Input: dimensioned drawing with shaded views. Units: mm. Origin: part minimum x, y, z. Round coordinates to 2 decimals unless told otherwise and drop trailing zeros. Loops run counter-clockwise (first coordinate to the right, second up) from the corner with the lowest first, then second, coordinate; pieces in that order, holes last. Notation, with made-up numbers: (34, -23) - (62, -23) arc R12 cw to (62, -16) - close; hole circle Ø1 at (22, 83). An arc over 180 degrees is marked (long way). Use CSV: the item, a comma, the result in double quotes. Start each with the question number.
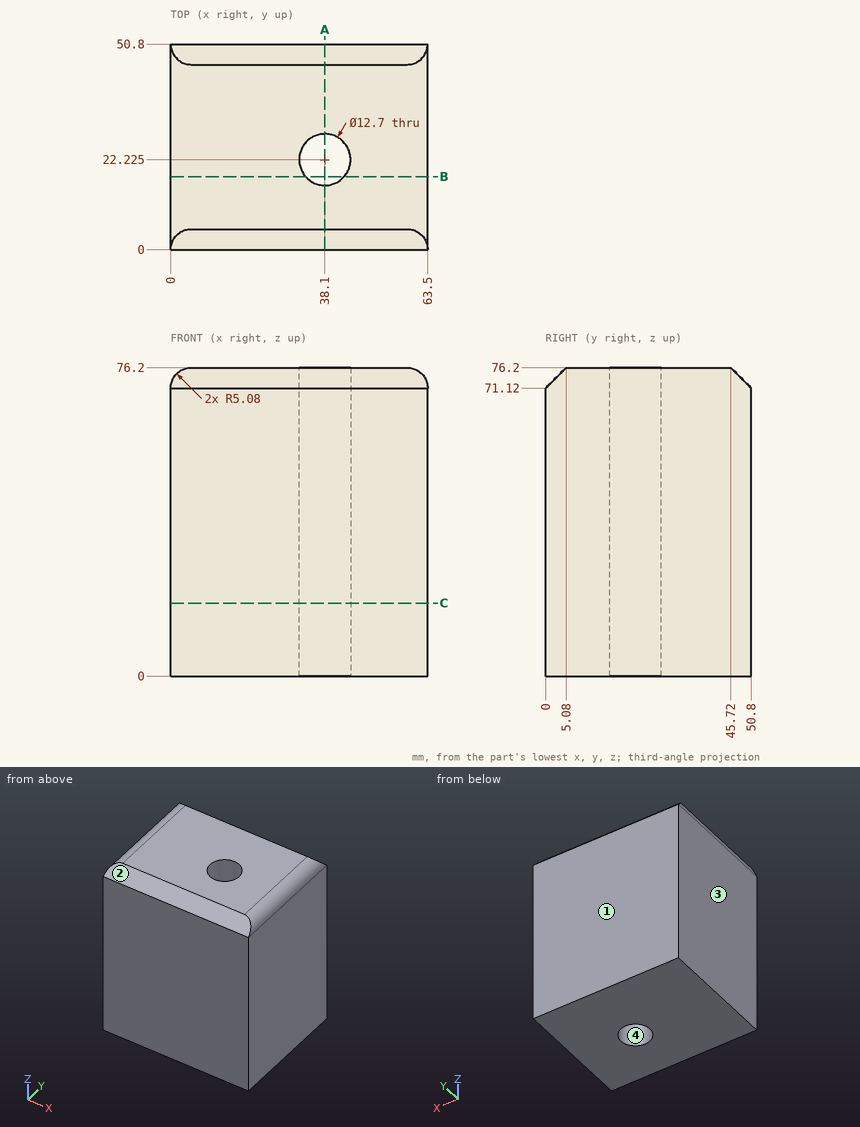
1. Mould query, pull axis Y, two halves, no side actions, for the marked faces 1, 2, 3 and 4. Classes: +Y half, -Y half, draft (parallel to the pull), parting line (faces both ways), or undercut.
2. Line query: line 1 along Y through (x, z) = (38.1, 45) (3 decimals); line 2 along X through (y, z) = (23, 40.5); line 3 along X through (y, z) = (28, 52). Output: solid intervals per line, ascending.
3. Section query C-C on z = 18. Return the cut outline in (x, y) (3 decimals), and give its area (3 significant figures).
4. Section query A-A on x = 38.1. Return the cut outline in (y, z) (3 decimals).
5. Section query B-B on y = 18. Return the cut outline in (x, z).
Values:
1,face 1,"+Y half"
1,face 2,"-Y half"
1,face 3,"draft"
1,face 4,"undercut"
2,line 1,"y = 0 to 15.875, 28.575 to 50.8"
2,line 2,"x = 0 to 31.8, 44.4 to 63.5"
2,line 3,"x = 0 to 35.46, 40.74 to 63.5"
3,outline,"(0, 0) - (63.5, 0) - (63.5, 50.8) - (0, 50.8) - close; hole circle Ø12.7 at (38.1, 22.225)"
3,area,"3,100 mm^2"
4,outline,"(0, 0) - (15.875, 0) - (15.875, 76.2) - (5.08, 76.2) - (0, 71.12) - close; (28.575, 0) - (50.8, 0) - (50.8, 71.12) - (45.72, 76.2) - (28.575, 76.2) - close"
5,outline,"(0, 0) - (33.36, 0) - (33.36, 76.2) - (5.08, 76.2) arc R5.08 ccw to (0, 71.12) - close; (42.84, 0) - (63.5, 0) - (63.5, 71.12) arc R5.08 ccw to (58.42, 76.2) - (42.84, 76.2) - close"
